from build123d import *

# Parameters (mm, degrees)
F1_DEPTH  = 8.5
F2_DEPTH  = 5
F3_R      = 2.6
F4_DEPTH  = 25
F5_R      = 2.6
F6_DEPTH  = 25
F7_SIZE   = 1
F8_W      = 6
F8_H      = 3
F9_DEPTH  = 1
F10_W     = 6
F10_H     = 3
F11_DEPTH = 1
F12_R     = 0.5


with BuildPart() as f1:
    # F0 (on Right) → F1 (new body, symmetric)
    with BuildSketch(Plane.YZ):
        Polygon((-0.3340116796, 1.9893845548), (-0.3340116796, -1.0106154452), (15.6659883204, -1.0106154452), (15.6659883204, 14.9893845548), (12.6659883204, 14.9893845548), (12.6659883204, 4.9893845548), (9.6659883204, 1.9893845548), align=None)
        Polygon((12.6659883204, 14.9893845548), (-0.3340116796, 1.9893845548), (9.6659883204, 1.9893845548), (12.6659883204, 4.9893845548), align=None)
    extrude(amount=F1_DEPTH, both=True)

    # F0 (on Right) → F2 (cut, symmetric)
    with BuildSketch(Plane.YZ):
        Polygon((12.6659883204, 14.9893845548), (-0.3340116796, 1.9893845548), (9.6659883204, 1.9893845548), (12.6659883204, 4.9893845548), align=None)
    extrude(amount=F2_DEPTH, both=True, mode=Mode.SUBTRACT)

    # F3 (on face) → F4 (cut)
    with BuildSketch(Plane.XZ.offset(-12.6659883204)):
        with Locations((0, 9.9893845548)):
            Circle(F3_R)
    extrude(amount=-F4_DEPTH, mode=Mode.SUBTRACT)

    # F5 (on face) → F6 (cut)
    with BuildSketch(Plane.XY.offset(1.9893845548)):
        with Locations((0, 4.6659883204)):
            Circle(F5_R)
    extrude(amount=-F6_DEPTH, mode=Mode.SUBTRACT)

    # F7
    f7_edges = [f1.edges().sort_by_distance(p)[0] for p in [
        (-8.5, 14.165988, 14.989385),
        (-8.5, 6.165988, 8.489385),
        (-8.5, -0.334012, 0.489385),
        (8.5, -0.334012, 0.489385),
        (8.5, 6.165988, 8.489385),
        (8.5, 14.165988, 14.989385),
        (-5, 11.165988, 3.489385),
        (5, 11.165988, 3.489385),
        (0, 15.665988, -1.010615),
    ]]
    chamfer(f7_edges, length=F7_SIZE)

    # F8 (on face) → F9 (join)
    with BuildSketch(Plane(origin=(0, 15.6659883204, 0), x_dir=(-1, 0, 0), z_dir=(0, 1, 0))):
        with Locations((0, 1.4893845548)):
            Rectangle(F8_W, F8_H)
    extrude(amount=F9_DEPTH)

    # F10 (on face) → F11 (join)
    with BuildSketch(Plane(origin=(0, 0, -1.0106154452), x_dir=(1, 0, 0), z_dir=(0, 0, -1))):
        with Locations((0, -13.1659883204)):
            Rectangle(F10_W, F10_H)
    extrude(amount=F11_DEPTH)

    # F12
    f12_edges = [f1.edges().sort_by_distance(p)[0] for p in [
        (3, 16.165988, 2.989385),
        (3, 16.165988, -0.010615),
        (-3, 16.165988, 2.989385),
        (-3, 16.165988, -0.010615),
        (-3, 11.665988, -1.510615),
        (-3, 14.665988, -1.510615),
        (3, 11.665988, -1.510615),
        (3, 14.665988, -1.510615),
    ]]
    fillet(f12_edges, radius=F12_R)


solid = f1.part
Check sheet for the modelled part. Datum: model origin and axes. Units: mm. A direction names the side the tool comes from. Coordinates: 2 decimals unless noted, no trailing zeros. Write each loop counter-clockwise with the first axis right and the second up, starting at its lowest first coordinate (ties: lowest second). Pieces come first, ordered by that corner, then holes.
Item 1: Cross-section at B-B on y = 7. Record the boundary of the cut face in (x, z).
Numbers:
outline: (-8.5, -1.01) - (-1.15, -1.01) - (-1.15, 1.99) - (-5, 1.99) - (-5, 9.32) - (-7.5, 9.32) - (-8.5, 7.91) - close; (1.15, -1.01) - (8.5, -1.01) - (8.5, 7.91) - (7.5, 9.32) - (5, 9.32) - (5, 1.99) - (1.15, 1.99) - close
Item 2: Depth check by flat-ended pin: pin 1 Ø3 at (x, y) = (-2.5, 6.5) entering from +Z; pin 2 Ø6 at (x, y) = (0, 4.67) entering from -Z; pin 3 Ø1.1 at (y, z) = (13.5, -2) entering from -X. Enter the tip coordinate at first touch or a pass-through.
Numbers:
pin 1: stops at z = 1.99
pin 2: stops at z = -1.01
pin 3: stops at x = -3
Item 3: Scan lines: probe 1 along Y at (x, z) = (0, 0.85); probe 2 along Z at (x, y) = (0, 13.3); probe 3 along X at (y, z) = (1.75, 2.5). Record each from-to range of solid material in increasing order.
Numbers:
probe 1: y = -0.33 to 2.07, 7.27 to 16.67
probe 2: z = -2.01 to 7.39, 12.59 to 14.99
probe 3: x = -8.5 to -5, 5 to 8.5
Item 4: Mould release check, pull along X, two halves, no side actions. Record for faces 1 (the face through (2, 7, -1.011)), 2 (the face through (-5, 8, 7)), 3 (the face through (8.007, 0.173, 0.51)): released by +X, released by -X, zero draft, split by the parting line, or undercut.
Numbers:
face 1: zero draft
face 2: undercut
face 3: released by +X
Item 5: Cross-section at D-D on x = 6.5. Record the boundary of the cut face in (y, z), then the cut area to 3 significant figures.
Numbers:
outline: (-0.33, -1.01) - (14.67, -1.01) - (15.67, -0.01) - (15.67, 14.99) - (12.67, 14.99) - (-0.33, 1.99) - close
area: 171 mm2
Item 6: Access from +Z, -Z, +X, -X, +Y, -Y to the whole of each face (thin tool, end or side, straight path). Record for faces 4 (the face through (-4.49, 10.79, 3.81)), 5 (the face through (6.268, 6.257, 8.58)), 6 (the face through (3, 16, 1)), 7 (the face through (0, 16, -0.011)), 8 (the face through (8.5, 10, 5)).
Numbers:
face 4: +Z, -Y
face 5: +Z, +X, -X, -Y
face 6: +Z, -Z, +X, +Y
face 7: -Z, +X, -X, +Y
face 8: +Z, -Z, +X, +Y, -Y
Item 7: Cross-section at C-C on z = 9.75. Record the boundary of the cut face in (x, y).
Numbers:
outline: (-8.5, 8.84) - (-7.5, 7.43) - (-5, 7.43) - (-5, 12.67) - (-2.59, 12.67) - (-2.59, 15.67) - (-8.5, 15.67) - close; (2.59, 12.67) - (5, 12.67) - (5, 7.43) - (7.5, 7.43) - (8.5, 8.84) - (8.5, 15.67) - (2.59, 15.67) - close
Item 8: Cross-section at A-A on x = 0. Record the boundary of the cut face in (y, z), then the cut area to 3 significant figures.
Numbers:
outline: (-0.33, -1.01) - (2.07, -1.01) - (2.07, 1.99) - (-0.33, 1.99) - close; (7.27, -1.01) - (11.67, -1.01) - (11.67, -2.01) - (14.67, -2.01) - (14.67, -1.01) - (15.67, -0.01) - (16.67, -0.01) - (16.67, 2.99) - (15.67, 2.99) - (15.67, 7.39) - (12.67, 7.39) - (12.67, 4.99) - (9.67, 1.99) - (7.27, 1.99) - close; (12.67, 12.59) - (15.67, 12.59) - (15.67, 14.99) - (12.67, 14.99) - close
area: 65.8 mm2
